Model file for the job. Use its own axes, mm. Face numbers are marked on the shaded views. A direction names the side the tool comes from. Give positions to 0.01 mm unless a question says otherwise; leave off trailing zeros. Write each loop counter-clockwise with the first axis right and the second up, starting at its lowest first coordinate (ties: lowest second). Pieces come first, ordered by that corner, then holes.
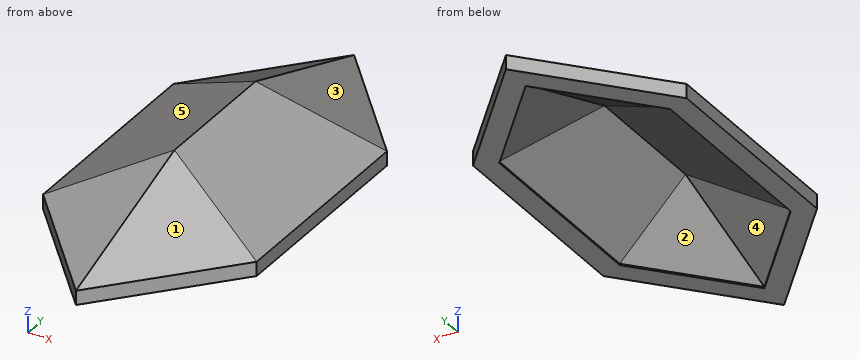
```python
from build123d import *

# Parameters (mm, degrees)
F0_W     = 7.62
F0_H     = 7.62
F1_DEPTH = 2.54
F2_SIZE2 = 3.80999
F2_SIZE  = 2.03199
F3_T     = -0.762


# Not quite as in the source:
# - a fillet or chamfer is up to 0.001 mm smaller than in the source, because OpenCascade refuses the exact size


with BuildPart() as f1:
    # F0 (on Top) → F1 (new body)
    with BuildSketch(Plane.XY):
        Rectangle(F0_W, F0_H)
        Polygon((-3.81, 3.81), (3.81, 3.81), (0, 8.1314574927), align=None)
        Polygon((0, -8.1314574927), (3.81, -3.81), (-3.81, -3.81), align=None)
    extrude(amount=F1_DEPTH)

    # F2 (size 2.032 and 3.81 in the source; OpenCascade refuses exactly that, so slightly less here)
    f2_edges = [f1.edges().sort_by_distance(p)[0] for p in [
        (3.81, 0, 2.54),
        (1.905, 5.970729, 2.54),
        (-1.905, -5.970729, 2.54),
        (-3.81, 0, 2.54),
        (-1.905, 5.970729, 2.54),
        (1.905, -5.970729, 2.54),
    ]]
    chamfer(f2_edges, length=F2_SIZE, length2=F2_SIZE2)

    # F3
    f3_openings = [f1.faces().sort_by_distance(p)[0] for p in [
        (0, 0, 0),
    ]]
    offset(amount=F3_T, openings=f3_openings)


solid = f1.part
```
1. Pull direction X, two halves, no side cores. Call the marked faces 3, 4 and 5: +X half, -X half, draft (parallel to the pull), parting line (faces both ways), or undercut.
Calculated:
face 3: +X half
face 4: undercut
face 5: -X half
2. Slice it at C-C, the plane x = -2.75. Write the cut outline in (y, z), and give its area (3 significant figures).
Calculated:
outline: (-5.01, 0) - (-3.86, 0) - (-3.86, 0.05) - (-3.41, 0.21) - (3.41, 0.21) - (3.86, 0.05) - (3.86, 0) - (5.01, 0) - (5.01, 0.51) - (3.41, 1.07) - (-3.41, 1.07) - (-5.01, 0.51) - close
area: 8.31 mm2
3. Pin check, flat tips, straight feed: P1, Ø1.5, axis at x = 1, y = 1.5, coming from the +Z side; P2, Ø1, axis at x = -1, z = 0.5, coming from the +Y side; P3, Ø1, axis at x = 1.5, y = -2, coming from the -Z side. Stop position of each tip, or through.
Calculated:
P1: stops at z = 2.41
P2: stops at y = 7.56
P3: stops at z = 0.61
4. Slice it at B-B, the plane z = 0.95. Write the cut outline in (x, y), and give its area (3 significant figures).
Calculated:
outline: (-2.98, -3.5) - (0, -6.88) - (2.98, -3.5) - (2.98, 3.5) - (0, 6.88) - (-2.98, 3.5) - close; hole (-1.36, -2.88) - (0, -4.43) - (1.36, -2.88) - (1.36, 2.88) - (0, 4.43) - (-1.36, 2.88) - close
area: 41.9 mm2
5. Slice it at D-D, the plane z = 2.25. Write the cut outline in (x, y).
Calculated:
outline: (-0.54, -2.58) - (0, -3.19) - (0.54, -2.58) - (0.54, 2.58) - (0, 3.19) - (-0.54, 2.58) - close
6. Probe probe 1 along X at (y, z) = (2, 1.5); probe 2 along X at (y, z) = (-4.5, 0.1); probe 3 along X at (y, z) = (-3.5, 1.5). List the from-to ranges inside material, lowest first.
Calculated:
probe 1: x = -1.95 to -0.33, 0.33 to 1.95
probe 2: x = -3.2 to -2.06, 2.06 to 3.2
probe 3: x = -1.6 to 1.6
7. Which spindle directions (+Z, -Z, +X, -X, +Y, -Y) get a long thin tool onto all of the face, cutting with end or side? Do the marked faces 1 and 2. Say none if no direction does.
Calculated:
face 1: +Z, +X, -Y
face 2: -Z
